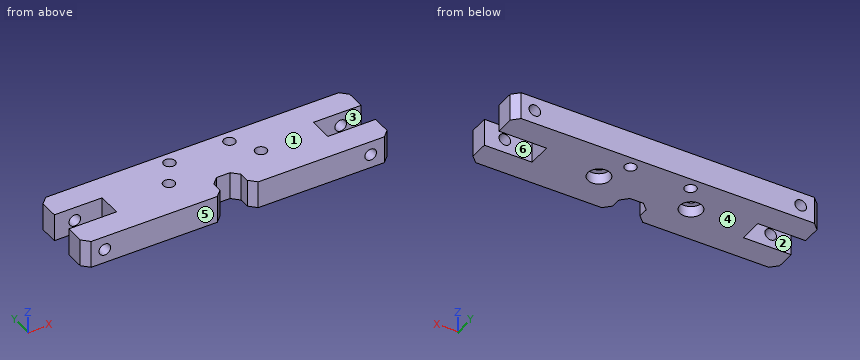
```python
from build123d import *

# Parameters (mm, degrees)
F1_DEPTH       = 8
F3_D           = 3.4
F4_D           = 3.4
F4_CBORE_D     = 6.5
F4_CBORE_DEPTH = 3.2
F6_D           = 3.4
F5_W           = 8
F5_H           = 7
F7_DEPTH       = 8
F8_SIZE        = 2


with BuildPart() as f1:
    # F0 (on Top) → F1 (new body)
    with BuildSketch(Plane.XY):
        Polygon((-45, -11), (45, -11), (45, -3.5), (31, -3.5), (31, 3.5), (45, 3.5), (45, 11), (-45, 11), (-45, 3.5), (-31, 3.5), (-31, -3.5), (-45, -3.5), align=None)
    extrude(amount=F1_DEPTH)

    # F3 (through all)
    with Locations(Plane.XZ.offset(11)):
        with Locations((-39, 4), (39, 4)):
            Hole(F3_D / 2)

    # F4 (through all)
    with Locations(Plane(origin=(0, 0, 0), x_dir=(1, 0, 0), z_dir=(0, 0, -1))):
        with Locations((-13.5, 0), (13.5, 0)):
            CounterBoreHole(F4_D / 2, F4_CBORE_D / 2, F4_CBORE_DEPTH)

    # F6 (through all)
    with Locations(Plane.XY.offset(8)):
        with Locations((-8.8, 7.5), (8.8, 7.5)):
            Hole(F6_D / 2)

    # F5 (on face) → F7 (cut, through all)
    with BuildSketch(Plane.XY.offset(8)):
        with Locations((0, -7.5)):
            Rectangle(F5_W, F5_H)
    extrude(amount=-F7_DEPTH, mode=Mode.SUBTRACT)

    # F8
    f8_edges = [f1.edges().sort_by_distance(p)[0] for p in [
        (-45, -11, 4),
        (45, -11, 4),
        (4, -11, 4),
        (4, -4, 4),
        (-4, -4, 4),
        (-4, -11, 4),
        (45, 11, 4),
        (-45, 11, 4),
    ]]
    chamfer(f8_edges, length=F8_SIZE)


solid = f1.part
```
For this review, take the finished solid that the model builds, in its own axes (mm). Face numbers are marked on the shaded views. A direction names the side the tool comes from. Coordinates: 2 decimals unless noted, no trailing zeros. Loops run counter-clockwise (first coordinate to the right, second up) from the corner with the lowest first, then second, coordinate; pieces in that order, holes last.
1. For line 1 (Y direction, x = 41.5, z = 3.25); line 2 (Z direction, x = 39, y = -7.75); line 3 (Y direction, x = -8.8, z = 1.75), list the stretches that pass through material, from the lowest coordinate up.
2. Add section C-C, the plane z = 1. Give the boundary of the cut face in (x, y).
3. Insertion check: P1, Ø2, axis at y = -1.5, z = 2.5, coming from the +X side; P2, Ø1, axis at y = -2.5, z = 5, coming from the -X side; P3, Ø5, axis at x = 13.5, y = 0, coming from the -Z side. Each pin has a flat end and moves straight along its axis. Give the tip position at first contact, or say it passes through.
4. Add section D-D, the plane x = -39. Give the boundary of the cut face in (y, z).
5. Mouldability with a two-part tool opening along Y and no side actions: class the marked faces 3, 4, 5 and 6 as +Y half, -Y half, draft (parallel to the pull), parting line (faces both ways), or undercut.
6. For the marked faces 1 and 2, list the 3-axis set-ups (+Z, -Z, +X, -X, +Y, -Y) from which the entire face can be reached by the end or side of a thin tool; tool diameter is ignored.
7. Add section A-A, the plane y = 7.5. Give the boundary of the cut face in (x, z).
8. Add section B-B, the plane x = -13.5. Give the boundary of the cut face in (y, z), then the cut area to 3 significant figures.
Result:
1. line 1: y = -11 to -3.5, 3.5 to 11
1. line 2: z = 0 to 2.3, 5.7 to 8
1. line 3: y = -11 to 5.8, 9.2 to 11
2. outline: (-45, -9) - (-43, -11) - (-6, -11) - (-4, -9) - (-4, -6) - (-2, -4) - (2, -4) - (4, -6) - (4, -9) - (6, -11) - (43, -11) - (45, -9) - (45, -3.5) - (31, -3.5) - (31, 3.5) - (45, 3.5) - (45, 9) - (43, 11) - (-43, 11) - (-45, 9) - (-45, 3.5) - (-31, 3.5) - (-31, -3.5) - (-45, -3.5) - close; hole circle Ø6.5 at (-13.5, 0); hole circle Ø3.4 at (-8.8, 7.5); hole circle Ø3.4 at (8.8, 7.5); hole circle Ø6.5 at (13.5, 0)
3. P1: stops at x = 31
3. P2: stops at x = -31
3. P3: stops at z = 3.2
4. outline: (-11, 0) - (-3.5, 0) - (-3.5, 2.3) - (-11, 2.3) - close; (-11, 5.7) - (-3.5, 5.7) - (-3.5, 8) - (-11, 8) - close; (3.5, 0) - (11, 0) - (11, 2.3) - (3.5, 2.3) - close; (3.5, 5.7) - (11, 5.7) - (11, 8) - (3.5, 8) - close
5. face 3: undercut
5. face 4: draft
5. face 5: -Y half
5. face 6: undercut
6. face 1: +Z, +X, -X, +Y, -Y
6. face 2: +Z, -Z, -X
7. outline: (-45, 0) - (-10.5, 0) - (-10.5, 8) - (-45, 8) - close; (-7.1, 0) - (7.1, 0) - (7.1, 8) - (-7.1, 8) - close; (10.5, 0) - (45, 0) - (45, 8) - (10.5, 8) - close; hole circle Ø3.4 at (-39, 4); hole circle Ø3.4 at (39, 4)
8. outline: (-11, 0) - (-3.25, 0) - (-3.25, 3.2) - (-1.7, 3.2) - (-1.7, 8) - (-11, 8) - close; (1.7, 3.2) - (3.25, 3.2) - (3.25, 0) - (11, 0) - (11, 8) - (1.7, 8) - close
8. area: 139 mm2
